Input: part model. Units: mm. Frame: model coordinates. A direction names the side the tool comes from. Give positions to 0.01 mm unless a question says otherwise; leave off trailing zeros. Loops run counter-clockwise (first coordinate to the right, second up) from the corner with the lowest first, then second, coordinate; pieces in that order, holes last. Notation, with made-up numbers: (75.5, -13) - (93.5, -13) arc R20 cw to (93.5, 4) - close; hole circle Ø7 at (80.5, 40). An arc over 180 degrees is marked (long way). One line per item, written item: value.
from build123d import *

# Parameters (mm, degrees)
PAD001_DEPTH  = 9
SKETCH005_R   = 5.5
SKETCH005_R_2 = 2
POCKET_DEPTH  = 2.6
CHAMFER_SIZE  = 2.5


with BuildPart() as part:
    # Sketch003 → Pad001 (new body, symmetric)
    with BuildSketch(Plane.XY):
        with BuildLine():
            ThreePointArc((-3.9577139867, -3.0555686868), (5, -2.4e-09), (-3.9577139837, 3.0555686906))
            ThreePointArc((-7.1239026623, 1.5), (-5.3600614281, 1.9098939553), (-3.9577139838, 3.0555686907))
            Line((-7.1239026623, 1.5), (-20, 1.5))
            Line((-20, -1.5), (-20, 1.5))
            Line((-20, -1.5), (-7.1239026639, -1.5))
            ThreePointArc((-3.9577139867, -3.0555686868), (-5.360061431, -1.9098939539), (-7.1239026639, -1.5))
        make_face()
    extrude(amount=PAD001_DEPTH, both=True)

    # Sketch005 → Pocket (cut, symmetric)
    with BuildSketch(Plane.XY.offset(4.25)):
        Circle(SKETCH005_R)
        Circle(SKETCH005_R_2, mode=Mode.SUBTRACT)
    pocket = extrude(amount=POCKET_DEPTH, both=True, mode=Mode.SUBTRACT)

    # Mirrored: Pocket across XY
    add(pocket.mirror(Plane.XY), mode=Mode.SUBTRACT)

    # Chamfer
    chamfer_edges = [part.edges().sort_by_distance(p)[0] for p in [
        (-2, 0, -6.85),
        (-2, 0, 1.65),
        (-2, 0, 6.85),
        (-2, 0, -1.65),
    ]]
    chamfer(chamfer_edges, length=CHAMFER_SIZE)


solid = part.part
Item 1: Section D-D, the plane z = -0.5. Output: boundary loops of the cut face in (x, y), and give its area (3 significant figures).
Verdict:
outline: (-20, -1.5) - (-7.12, -1.5) arc R4 cw to (-3.96, -3.06) arc R5 ccw (long way) to (-3.96, 3.06) arc R4 cw to (-7.12, 1.5) - (-20, 1.5) - close
area: 125 mm^2
Item 2: Section C-C, the plane x = 0. Output: boundary loops of the cut face in (y, z), and give its area (3 significant figures).
Verdict:
outline: (-5, -9) - (5, -9) - (5, -6.85) - (4.5, -6.85) - (2, -4.35) - (2, -4.15) - (4.5, -1.65) - (5, -1.65) - (5, 1.65) - (4.5, 1.65) - (2, 4.15) - (2, 4.35) - (4.5, 6.85) - (5, 6.85) - (5, 9) - (-5, 9) - (-5, 6.85) - (-4.5, 6.85) - (-2, 4.35) - (-2, 4.15) - (-4.5, 1.65) - (-5, 1.65) - (-5, -1.65) - (-4.5, -1.65) - (-2, -4.15) - (-2, -4.35) - (-4.5, -6.85) - (-5, -6.85) - close
area: 143 mm^2
Item 3: Section A-A, the plane z = -5.5. Output: boundary loops of the cut face in (x, y).
Verdict:
outline: (-20, -1.5) - (-7.12, -1.5) arc R4 cw to (-5.1, -2.05) arc R5.5 cw to (-5.1, 2.05) arc R4 cw to (-7.12, 1.5) - (-20, 1.5) - close; circle Ø6.3 at (0, 0)
Item 4: Access query for faces 1 (the face through (-14, -1.5, 0)), 2 (the face through (-5.5, 0, -4.3)), 3 (the face through (-20, 0, 0)), 4 (the face through (-13, 1.5, 0)). Directions: +Z, -Z, +X, -X, +Y, -Y. A direction counts if a zero-diameter tool reaches every point of the face in a straight line with its end or side. Return the directions, or none.
Verdict:
face 1: +Z, -Z, -X, -Y
face 2: none
face 3: +Z, -Z, -X, +Y, -Y
face 4: +Z, -Z, -X, +Y
Item 5: Section B-B, the plane y = 0. Output: boundary loops of the cut face in (x, z).
Verdict:
outline: (-20, -9) - (5, -9) - (5, -6.85) - (4.5, -6.85) - (2, -4.35) - (2, -4.15) - (4.5, -1.65) - (5, -1.65) - (5, 1.65) - (4.5, 1.65) - (2, 4.15) - (2, 4.35) - (4.5, 6.85) - (5, 6.85) - (5, 9) - (-20, 9) - close; hole (-5.5, -6.85) - (-4.5, -6.85) - (-2, -4.35) - (-2, -4.15) - (-4.5, -1.65) - (-5.5, -1.65) - close; hole (-5.5, 1.65) - (-4.5, 1.65) - (-2, 4.15) - (-2, 4.35) - (-4.5, 6.85) - (-5.5, 6.85) - close
Item 6: Pin query (flat end, axial travel): P1, Ø4, axis at x = -12, z = 0.5, coming from the -Y side; P2, Ø1.5, axis at x = -17, y = 2.5, coming from the -Z side; P3, Ø10.5, axis at x = -10.5, z = -3, coming from the +Y side. Return the tip coordinate at first contact, or that it passes through.
Verdict:
P1: stops at y = -1.5
P2: passes through
P3: stops at y = 1.97
Item 7: Draft query along X for faces 5 (the face through (-5.76, 1.74, 0.13)), 6 (the face through (5, 0, 8)), 7 (the face through (-5, 0, -6.85)). Return one class per face: pulls with the +X half, pulls with the -X half, needs draft (parallel to the pull), parting line crosses it, or undercut.
Verdict:
face 5: pulls with the -X half
face 6: parting line crosses it
face 7: undercut
Item 8: Material intervals for L1, parallel to Z at x = 2.25, y = 0.5; L2, parallel to Z at x = -3, y = -2.5; L3, parallel to Y at x = -15.5, z = -3, sorted ascending.
Verdict:
L1: z = -9 to -4.65, -3.85 to 3.85, 4.65 to 9
L2: z = -9 to -6.26, -2.24 to 2.24, 6.26 to 9
L3: y = -1.5 to 1.5
